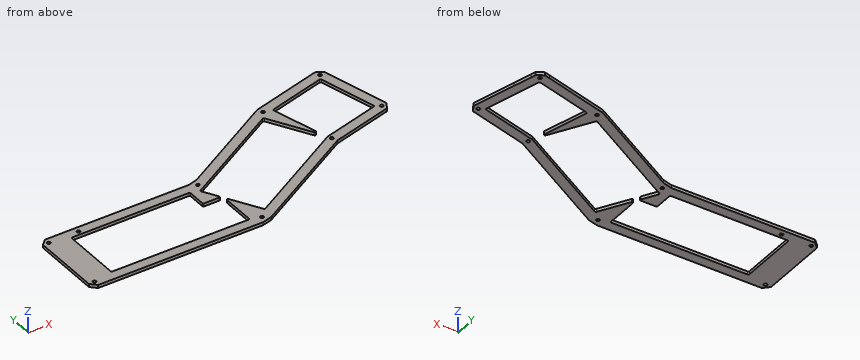
from build123d import *

# Parameters (mm, degrees)
ESQUISSE1_R        = 1.6
BOSS_EXTRU_1_DEPTH = 3


with BuildPart() as part:
    # Esquisse1 → Boss.-Extru.1 (new body)
    with BuildSketch(Plane.XY):
        Polygon((-75.988646329, 49.585106383), (-95.960869343, 49.585106383), (-101.253762562, 44.292213164), (-101.253762562, 35.79522772), (-101.253762562, -22.122000398), (-95.960869343, -27.414893617), (63.734552111, -27.414893617), (73.191845678, -24.880819443), (177.743787613, 35.482272378), (236.017194438, 51.096584676), (239.759835125, 57.579028501), (228.577013006, 99.31388882), (223.918643626, 116.699160027), (222.600104344, 121.736116557), (216.144691957, 125.488029577), (211.058449045, 124.125174896), (148.022896982, 107.234849626), (52.44172146, 52.051032209), (43.238760989, 49.585106383), align=None)
        with Locations((-95.753762562, 44.085106383)):
            Circle(ESQUISSE1_R, mode=Mode.SUBTRACT)
        with Locations((-66.988646329, 44.085106383)):
            Circle(ESQUISSE1_R, mode=Mode.SUBTRACT)
        with Locations((-95.753762562, -21.914893617)):
            Circle(ESQUISSE1_R, mode=Mode.SUBTRACT)
        with Locations((67.039694146, -20.835264486)):
            Circle(ESQUISSE1_R, mode=Mode.SUBTRACT)
        with Locations((49.263745973, 45.505477252)):
            Circle(ESQUISSE1_R, mode=Mode.SUBTRACT)
        with Locations((150.12930694, 102.149526137)):
            Circle(ESQUISSE1_R, mode=Mode.SUBTRACT)
        with Locations((217.363403759, 120.120565138)):
            Circle(ESQUISSE1_R, mode=Mode.SUBTRACT)
        with Locations((234.393639901, 56.355573542)):
            Circle(ESQUISSE1_R, mode=Mode.SUBTRACT)
        with Locations((175.637377655, 40.567595866)):
            Circle(ESQUISSE1_R, mode=Mode.SUBTRACT)
        with BuildLine():
            Line((-76.753762562, 39.085106383), (-76.753762562, -16.914893617))
            ThreePointArc((-76.753762562, -16.914893617), (-76.460869343, -17.622000398), (-75.753762562, -17.914893617))
            Line((-75.753762562, -17.914893617), (56.011353671, -17.914893617))
            ThreePointArc((56.011353671, -17.914893617), (56.718460453, -17.622000398), (57.011353671, -16.914893617))
            Line((57.011353671, -16.914893617), (57.011353671, 14.621004768))
            ThreePointArc((57.011353671, 14.621004768), (57.752534626, 15.586930594), (58.877379075, 15.121004768))
            Line((58.877379075, 15.121004768), (74.527293708, -11.98544251))
            ThreePointArc((74.527293708, -11.98544251), (75.134500067, -12.451368337), (75.893319112, -12.351467914))
            Line((75.893319112, -12.351467914), (174.076924484, 44.334863077))
            Line((174.076924484, 44.334863077), (228.528734589, 58.925181621))
            ThreePointArc((228.528734589, 58.925181621), (229.135940948, 59.391107448), (229.235841371, 60.149926493))
            Line((229.235841371, 60.149926493), (214.741974845, 114.241772765))
            ThreePointArc((214.741974845, 114.241772765), (214.276049019, 114.848979124), (213.517229973, 114.948879546))
            Line((213.517229973, 114.948879546), (159.425383701, 100.45501302))
            ThreePointArc((159.425383701, 100.45501302), (158.818177343, 99.989087194), (158.71827692, 99.230268149))
            Line((158.71827692, 99.230268149), (170.271736655, 56.112169417))
            ThreePointArc((170.271736655, 56.112169417), (169.688494261, 54.929470839), (168.439785425, 55.353350371))
            Line((168.439785425, 55.353350371), (146.120215143, 94.011980101))
            ThreePointArc((146.120215143, 94.011980101), (145.513008785, 94.477905928), (144.75418974, 94.378005505))
            Line((144.75418974, 94.378005505), (46.893319112, 37.878005505))
            ThreePointArc((46.893319112, 37.878005505), (46.427393286, 37.270799147), (46.527293708, 36.511980101))
            Line((46.527293708, 36.511980101), (54.567977999, 22.585106383))
            ThreePointArc((54.567977999, 22.585106383), (54.567977999, 21.585106383), (53.701952595, 21.085106383))
            Line((53.701952595, 21.085106383), (39.011353671, 21.085106383))
            ThreePointArc((39.011353671, 21.085106383), (38.30424689, 21.377999602), (38.011353671, 22.085106383))
            Line((38.011353671, 22.085106383), (38.011353671, 39.085106383))
            ThreePointArc((38.011353671, 39.085106383), (37.718460453, 39.792213164), (37.011353671, 40.085106383))
            Line((37.011353671, 40.085106383), (-75.753762562, 40.085106383))
            ThreePointArc((-75.753762562, 40.085106383), (-76.460869343, 39.792213164), (-76.753762562, 39.085106383))
        make_face(mode=Mode.SUBTRACT)
    extrude(amount=BOSS_EXTRU_1_DEPTH)


solid = part.part
For this review, take the finished solid that the model builds, in its own axes (mm). Round coordinates to 2 decimals unless told otherwise and drop trailing zeros. Loops run counter-clockwise (first coordinate to the right, second up) from the corner with the lowest first, then second, coordinate; pieces in that order, holes last. Notation, with made-up numbers: (14.5, 65.5) - (21.5, 65.5) arc R27 cw to (21.5, 93.5) - close; hole circle Ø3 at (22, 86). An arc over 180 degrees is marked (long way). Use one line per item in the form item = value.
Item 1: Consider section A-A on x = 30. Write out the cut boundary in (y, z), then the cut area to 3 significant figures.
Answers:
outline = (-27.41, 0) - (-17.91, 0) - (-17.91, 3) - (-27.41, 3) - close; (40.09, 0) - (49.59, 0) - (49.59, 3) - (40.09, 3) - close
area = 57.0 mm^2
Item 2: Consider section D-D on x = 125.5. Write out the cut boundary in (y, z), then the cut area to 3 significant figures.
Answers:
outline = (5.32, 0) - (16.29, 0) - (16.29, 3) - (5.32, 3) - close; (83.26, 0) - (94.23, 0) - (94.23, 3) - (83.26, 3) - close
area = 65.8 mm^2
Item 3: For line 1 (Y direction, x = -6.5, z = 0.95); line 2 (X direction, y = 83, z = 2.65); line 3 (X direction, y = -3, z = 1.25), list the stretches that pass through material, from the lowest coordinate up.
Answers:
line_1 = -27.41 to -17.91, 40.09 to 49.59
line_2 = 106.05 to 125.05, 152.48 to 163.07, 223.11 to 232.95
line_3 = -101.25 to -76.75, 57.01 to 69.34, 92.09 to 111.09
Item 4: Consider section B-B on y = 84. Write out the cut boundary in (x, z).
Answers:
outline = (107.78, 0) - (126.78, 0) - (126.78, 3) - (107.78, 3) - close; (151.9, 0) - (162.8, 0) - (162.8, 3) - (151.9, 3) - close; (222.85, 0) - (232.68, 0) - (232.68, 3) - (222.85, 3) - close
Item 5: Clearance check with flat-ended pins moving along their axes: P1, Ø1.5, axis at y = 7, z = 1, coming from the +X side; P2, Ø1.5, axis at x = -34.5, z = 1.5, coming from the +Y side. State where each tip first meets the part, or that it passes through.
Answers:
P1 = 129.71
P2 = 49.59
Item 6: Consider section C-C on y = 5. Write out the cut boundary in (x, z), then the cut area to 3 significant figures.
Answers:
outline = (-101.25, 0) - (-76.75, 0) - (-76.75, 3) - (-101.25, 3) - close; (57.01, 0) - (64.72, 0) - (64.72, 3) - (57.01, 3) - close; (105.95, 0) - (124.95, 0) - (124.95, 3) - (105.95, 3) - close
area = 154 mm^2
